Read the model definition and answer for the solid it produces. Units are mm, in the model's axes. A direction names the side the tool comes from. Coordinates: 2 decimals unless noted, no trailing zeros. Order: outer loops, then holes, each group sorted by start corner. A loop starts at its lowest first (then second) coordinate and runs counter-clockwise, first axis right, second up. Notation, with made-up numbers: M -7,16.25 L 6,16.25 A28 ccw 6,37.25 Z; hole C 88,59.25 d10. An arc over 180 degrees is marked long. Write each question's results on one line, items separated by ' | '.
```python
from build123d import *

# Parameters (mm, degrees)
SKETCH1_R           = 1.6
BOSS_EXTRUDE1_DEPTH = 3
SKETCH6_W           = 10.163490601
SKETCH6_H           = 3.2
SKETCH6_W_2         = 8.2
SKETCH6_W_3         = 3.2
SKETCH6_H_2         = 5.2
CUT_EXTRUDE4_DEPTH  = 4


with BuildPart() as part:
    # Sketch1 → Boss-Extrude1 (new body)
    with BuildSketch(Plane(origin=(0, 0, 0), x_dir=(1, 0, 0), z_dir=(0, 1, 0))):
        with BuildLine():
            Line((21.058452488, 3.842990858), (17.188733854, 5.16651258))
            Line((17.188733854, 5.16651258), (17.188733854, 6.83348742))
            Line((17.188733854, 6.83348742), (21.058452488, 8.157009142))
            Line((21.058452488, 8.157009142), (21.058452488, 9.842990858))
            Line((21.058452488, 9.842990858), (17.188733854, 11.16651258))
            Line((17.188733854, 11.16651258), (17.188733854, 12.83348742))
            Line((17.188733854, 12.83348742), (21.058452488, 14.157009142))
            Line((21.058452488, 14.157009142), (21.058452488, 15.842990858))
            Line((21.058452488, 15.842990858), (17.188733854, 17.16651258))
            Line((17.188733854, 17.16651258), (17.188733854, 18.83348742))
            Line((17.188733854, 18.83348742), (21.058452488, 20.157009142))
            Line((21.058452488, 20.157009142), (21.058452488, 21.842990858))
            Line((21.058452488, 21.842990858), (17.188733854, 23.16651258))
            Line((17.188733854, 23.16651258), (17.188733854, 24.83348742))
            Line((17.188733854, 24.83348742), (21.058452488, 26.157009142))
            Line((21.058452488, 26.157009142), (21.058452488, 27.842990858))
            Line((21.058452488, 27.842990858), (17.188733854, 29.16651258))
            Line((17.188733854, 29.16651258), (17.188733854, 30.83348742))
            Line((17.188733854, 30.83348742), (21.058452488, 32.157009142))
            Line((21.058452488, 32.157009142), (21.058452488, 33.842990858))
            Line((21.058452488, 33.842990858), (17.188733854, 35.16651258))
            Line((17.188733854, 35.16651258), (17.188733854, 36.83348742))
            Line((17.188733854, 36.83348742), (21.058452488, 38.157009142))
            Line((21.058452488, 38.157009142), (21.058452488, 39.842990858))
            Line((21.058452488, 39.842990858), (17.188733854, 41.16651258))
            Line((17.188733854, 41.16651258), (17.188733854, 42.83348742))
            Line((17.188733854, 42.83348742), (21.058452488, 44.157009142))
            Line((21.058452488, 44.157009142), (21.058452488, 45.842990858))
            Line((21.058452488, 45.842990858), (17.188733854, 47.16651258))
            Line((17.188733854, 47.16651258), (17.188733854, 48.83348742))
            Line((17.188733854, 48.83348742), (21.058452488, 50.157009142))
            Line((21.058452488, 50.157009142), (21.058452488, 51.842990858))
            Line((21.058452488, 51.842990858), (17.188733854, 53.16651258))
            Line((17.188733854, 53.16651258), (17.188733854, 54.83348742))
            Line((17.188733854, 54.83348742), (21.058452488, 56.157009142))
            Line((21.058452488, 56.157009142), (21.058452488, 57.842990858))
            Line((21.058452488, 57.842990858), (17.188733854, 59.16651258))
            Line((17.188733854, 59.16651258), (17.188733854, 60.83348742))
            Line((17.188733854, 60.83348742), (21.058452488, 62.157009142))
            Line((21.058452488, 62.157009142), (21.058452488, 62.842990858))
            ThreePointArc((21.058452488, 62.842990858), (21.351345707, 63.550097639), (22.058452488, 63.842990858))
            Line((22.058452488, 63.842990858), (45.872217102, 63.842990858))
            ThreePointArc((45.872217102, 63.842990858), (49.407751008, 62.378524764), (50.872217102, 58.842990858))
            Line((50.872217102, 58.842990858), (50.872217102, -34.901443346))
            ThreePointArc((50.872217102, -34.901443346), (49.407751008, -38.436977252), (45.872217102, -39.901443346))
            Line((45.872217102, -39.901443346), (-45.872217102, -39.901443346))
            ThreePointArc((-45.872217102, -39.901443346), (-49.407751008, -38.436977252), (-50.872217102, -34.901443346))
            Line((-50.872217102, -34.901443346), (-50.872217102, 58.842990858))
            ThreePointArc((-50.872217102, 58.842990858), (-49.407751008, 62.378524764), (-45.872217102, 63.842990858))
            Line((-45.872217102, 63.842990858), (-26.058452488, 63.842990858))
            ThreePointArc((-26.058452488, 63.842990858), (-22.522918582, 62.378524764), (-21.058452488, 58.842990858))
            Line((-21.058452488, 58.842990858), (-21.058452488, -3.842990858))
            ThreePointArc((-21.058452488, -3.842990858), (0, -24.901443346), (21.058452488, -3.842990858))
            Line((21.058452488, -3.842990858), (21.058452488, -2.157009142))
            Line((21.058452488, -2.157009142), (17.188733854, -0.83348742))
            Line((17.188733854, -0.83348742), (17.188733854, 0.83348742))
            Line((17.188733854, 0.83348742), (21.058452488, 2.157009142))
            Line((21.058452488, 2.157009142), (21.058452488, 3.842990858))
        make_face()
        with Locations((26.558452488, -14.587678732)):
            Circle(SKETCH1_R, mode=Mode.SUBTRACT)
        with Locations((-26.558452488, -14.587678732)):
            Circle(SKETCH1_R, mode=Mode.SUBTRACT)
        with Locations((-26.558452488, 38.529226244)):
            Circle(SKETCH1_R, mode=Mode.SUBTRACT)
        with Locations((26.558452488, 38.529226244)):
            Circle(SKETCH1_R, mode=Mode.SUBTRACT)
    extrude(amount=BOSS_EXTRUDE1_DEPTH)

    # Sketch6 → Cut-Extrude4 (cut, through all)
    with BuildSketch(Plane(origin=(0, 0, 0), x_dir=(1, 0, 0), z_dir=(0, 1, 0))):
        with Locations((9.963490601, -38.401443346)):
            Rectangle(SKETCH6_W, SKETCH6_H)
        with Locations((29.890471802, -38.401443346)):
            Rectangle(SKETCH6_W, SKETCH6_H)
        with Locations((-29.890471802, -38.401443346)):
            Rectangle(SKETCH6_W, SKETCH6_H)
        with Locations((-9.963490601, -38.401443346)):
            Rectangle(SKETCH6_W, SKETCH6_H)
        with Locations((-30.872217102, 45.342990858)):
            Rectangle(SKETCH6_W_2, SKETCH6_H)
        with Locations((33.372217102, -27.401443346)):
            Rectangle(SKETCH6_W_3, SKETCH6_H_2)
        Polygon((34.972217102, 41.742990858), (34.972217102, 46.942990858), (26.772217102, 46.942990858), (26.772217102, 43.742990858), (31.772217102, 43.742990858), (31.772217102, 41.742990858), align=None)
        with Locations((18.372217102, -27.401443346)):
            Rectangle(SKETCH6_W_3, SKETCH6_H_2)
    extrude(amount=CUT_EXTRUDE4_DEPTH, mode=Mode.SUBTRACT)


solid = part.part
```
(1) Given pin 1 (0.9 mm diameter, centred on y = 1.5, z = 39, fed in from -X); pin 2 (2 mm diameter, centred on x = -19.5, z = 4, fed in from -Y), each flat-ended and moving along its own axis, determine where each tip first touches the part or whether it passes through.
Conclusion:
pin 1: x = -49.29 | pin 2: through
(2) The mould has two halves that part along Z. Classify faces 1 (the flat face through (34.972, 1, 38)), 2 (the flat face through (19.097, 1.479, -31.486)), 3 (the flat face through (-10, 1, 36.801)): pulls with the +Z half, pulls with the -Z half, needs draft (parallel to the pull), parting line crosses it, or undercut.
Conclusion:
face 1: needs draft | face 2: undercut | face 3: pulls with the +Z half
(3) The part is cut by section C-C, the plane y = 2.35. Count the separate pieces of the cut face and the enclosed holes in it, then the cut area to 3 significant figures.
Conclusion:
separate pieces: 1 | enclosed holes: 8 | area: 6,860 mm²
(4) For faces 4 (the flat face through (19.151, 1.479, -52.495)), 5 (the flat face through (23, 0, -13)), 6 (the flat face through (10, 1, 36.801)), determine the directions among +Z, -Z, +X, -X, +Y, -Y from which every point of the face is accessible in a straight line to the end or side of a thin tool.
Conclusion:
face 4: +Y, -Y | face 5: +Z, -Z, +X, -X, -Y | face 6: +Z, +Y, -Y
(5) Straight lines are drawn through the part: line 1 (X direction, y = 1, z = 27); line 2 (X direction, y = 1.5, z = -42.5); line 3 (X direction, y = 2.8, z = -15.5). For each, find the intervals that lie inside material, in ascending order.
Conclusion:
line 1: -50.87 to 16.77, 19.97 to 31.77, 34.97 to 50.87 | line 2: -50.87 to -21.06, 17.19 to 31.77, 34.97 to 50.87 | line 3: -50.87 to -21.06, 21.06 to 50.87
(6) The part is cut by section A-A, the plane z = 19. Write down the section's boundary in (x, y).
Conclusion:
outline: M -50.87,0 L -14.62,0 L -14.62,3 L -50.87,3 Z; M 14.62,0 L 50.87,0 L 50.87,3 L 14.62,3 Z
(7) The part is cut by section B-B, the plane x = 0. Write down the section's boundary in (y, z).
Conclusion:
outline: M 0,24.9 L 3,24.9 L 3,39.9 L 0,39.9 Z
